Geometry check sheet. Reference: the model listing, model coordinates, mm. Face numbers are marked on the shaded views. A direction names the side the tool comes from. Round coordinates to 2 decimals unless told otherwise and drop trailing zeros. Order: outer loops, then holes, each group sorted by start corner. A loop starts at its lowest first (then second) coordinate and runs counter-clockwise, first axis right, second up. Notation, with made-up numbers: M 62.5,33.25 L 67.5,33.25 A18 ccw 67.5,64.25 Z; hole C -8,-18 d10. An arc over 180 degrees is marked long. Answer as a JSON object with one key per item and string values. Group by question number.
```python
from build123d import *
from build123d import SkipClean  # not in build123d's __all__

# Parameters (mm, degrees)
F0_W          = 151.5855640173
F0_H          = 149.6286615729
F1_DEPTH      = 11.684
F2_DEPTH      = 25.4
F3_W          = 4.1966233402
F3_H          = 25.7666455582
F3_W_2        = 24.8086545616
F3_H_2        = 24.7343285009
F3_W_3        = 8.3932466805
F3_H_3        = 20.2822238207
F3_W_4        = 29.5776501298
F3_H_4        = 8.4610134363
F5_DEPTH      = 25.4
F6_DEPTH      = 25.4
F8_W          = 13.618723955
F8_H          = 11.8162455037
F9_DEPTH      = 88.646
F10_W         = 90.7247327268
F10_H         = 75.9043544531
F11_DEPTH     = 13.97
F13_DEPTH     = 25.4
F14_DEPTH     = 125.476
F16_DEPTH     = 25.4
F17_R         = 4.969033059
F18_DEPTH     = 117.348
F20_DEPTH     = 87.376
F21_R         = 6.1087740457
F22_DEPTH     = 25.4
F23_DEPTH     = 25.4
F24_DEPTH     = 25.4
F25_R         = 5.08
F26_T1_DEPTH  = 44.704
F26_S5_W      = 5.08
F26_S5_H      = 5.08
F26_T6_DEPTH  = 5.08
F26_S11_W     = 5.08
F26_S11_H     = 5.08
F26_T12_DEPTH = 5.08
F27_W         = 27.1943286061
F27_H         = 16.5108405054
F28_DEPTH     = 61.722
F29_DEPTH     = 25.4
F30_DEPTH     = 160.02
F31_DEPTH     = 46.482


# Not quite as in the source:
# - a fillet or chamfer that OpenCascade refuses, or shapes differently, is made with other operations: its cross-section is extruded or revolved along the edge and cut away or added
# - after a boolean that leaves OpenCascade's solid faulty, fix() repairs it
# - a feature names something its author has since deleted; it is built from what else it names


with BuildPart() as f1:
    # F0 (on Top) → F1 (new body)
    with BuildSketch(Plane.XY):
        with Locations((1.5608146787, -0.5317740142)):
            Rectangle(F0_W, F0_H)
    extrude(amount=F1_DEPTH)

    # F2 (add): a face of the model
    f2_faces = [f1.faces().sort_by_distance(p)[0] for p in [
        (1.5608146787, -0.5317740142, 0),
    ]]
    extrude(f2_faces, amount=F2_DEPTH)

    # F3 (on face) → F5 (join)
    with BuildSketch(Plane(origin=(0, 0, -25.4), x_dir=(1, 0, 0), z_dir=(0, 0, -1))):
        with Locations((45.1576719061, 3.9362064563)):
            Rectangle(F3_W, F3_H)
        with Locations((-27.7178613469, -21.3142805733)):
            Rectangle(F3_W_2, F3_H_2)
        with Locations((47.2559835762, -43.8225567341)):
            Rectangle(F3_W_3, F3_H_3)
        with Locations((-54.0488772094, 67.9751783609)):
            Rectangle(F3_W_4, F3_H_4)
    extrude(amount=F5_DEPTH)

    # F6 (add): faces of the model
    f6_faces = [f1.faces().sort_by_distance(p)[0] for p in [
        (-54.0488772094, -67.9751783609, -50.8),
        (-27.7178613469, 21.3142805733, -50.8),
        (45.1576719061, -3.9362064563, -50.8),
        (47.2559835762, 43.8225567341, -50.8),
    ]]
    extrude(f6_faces, amount=F6_DEPTH)

    # F8 (on face) → F9 (join)
    with BuildSketch(Plane.XY.offset(11.684)):
        with Locations((-1.9266440067, -0.4005506635)):
            Rectangle(F8_W, F8_H)
    extrude(amount=F9_DEPTH)

    # F10 (on face) → F11 (join)
    with BuildSketch(Plane.XY.offset(100.33)):
        with Locations((-2.2270549089, -2.4033039808)):
            Rectangle(F10_W, F10_H)
    extrude(amount=F11_DEPTH)

    # F12 (on face) → F13 (join)
    with BuildSketch(Plane.XZ.offset(40.3554812074)):
        with BuildLine():
            ThreePointArc((-2.2270549227, 100.33), (2.7120859528, 102.3758591285), (4.7579450911, 107.315))
            ThreePointArc((4.7579450911, 107.315), (2.712085945, 112.2541408793), (-2.227054945, 114.3))
            ThreePointArc((-2.227054945, 114.3), (-9.2120549089, 107.3149999888), (-2.2270549227, 100.33))
        make_face()
    extrude(amount=F13_DEPTH)

    # F14 (add): a face of the model
    f14_faces = [f1.faces().sort_by_distance(p)[0] for p in [
        (-2.2270549089, -65.7554812074, 107.315),
    ]]
    with SkipClean():  # cleaning this boolean's faces spoils the solid; the shape is the same uncleaned
        extrude(f14_faces, amount=F14_DEPTH)

    # F15 (on face) → F16 (join)
    with BuildSketch(Plane.YZ.offset(43.1353114545)):
        with BuildLine():
            Line((-1.1355586467, 114.3), (1.1355586467, 114.3))
            ThreePointArc((1.1355586467, 114.3), (0, 114.4064722454), (-1.1355586467, 114.3))
        make_face()
        with BuildLine():
            ThreePointArc((-1.1355586467, 114.3), (-3.8974510358, 103.5937641266), (6.1087740457, 108.2976981997))
            ThreePointArc((6.1087740457, 108.2976981997), (4.7039340732, 112.1951492356), (1.1355586467, 114.3))
            Line((1.1355586467, 114.3), (-1.1355586467, 114.3))
        make_face()
    extrude(amount=F16_DEPTH)

    add(f1.part.fix(), mode=Mode.REPLACE)

    # F17 (on face) → F18 (join)
    with BuildSketch(Plane(origin=(0, 35.5488732457, 0), x_dir=(-1, 0, 0), z_dir=(0, 1, 0))):
        with Locations((0, 105.8959811926)):
            Circle(F17_R)
    extrude(amount=F18_DEPTH)

    # F19 (on face) → F20 (join)
    with BuildSketch(Plane(origin=(-47.5894212723, 0, 0), x_dir=(0, -1, 0), z_dir=(-1, 0, 0))):
        with BuildLine():
            Line((-3.5482673546, 114.3), (3.5482673546, 114.3))
            ThreePointArc((3.5482673546, 114.3), (0, 115.3617326707), (-3.5482673546, 114.3))
        make_face()
        with BuildLine():
            ThreePointArc((-3.5482673546, 114.3), (-3.0667012813, 103.2161631583), (6.4599488467, 108.901783824))
            ThreePointArc((6.4599488467, 108.901783824), (5.6856206657, 111.9684851053), (3.5482673546, 114.3))
            Line((3.5482673546, 114.3), (-3.5482673546, 114.3))
        make_face()
    extrude(amount=F20_DEPTH)

    # F21 (on face) → F22 (join)
    with BuildSketch(Plane.YZ.offset(68.5353114545)):
        with Locations((0, 108.2976981997)):
            Circle(F21_R)
    extrude(amount=F22_DEPTH)

    # F23 (add): faces of the model
    f23_faces = [f1.faces().sort_by_distance(p)[0] for p in [
        (0, 152.8968732457, 105.8959811926),
        (-2.2270549089, -191.2314812074, 107.315),
    ]]
    extrude(f23_faces, amount=F23_DEPTH, dir=(0, 1, 0))

    # F24 (add): a face of the model
    f24_faces = [f1.faces().sort_by_distance(p)[0] for p in [
        (93.9353114545, 0, 108.2976981997),
    ]]
    extrude(f24_faces, amount=F24_DEPTH)

    # F25
    f25_edges = [f1.edges().sort_by_distance(p)[0] for p in [
        (77.353597, -0.531774, 11.684),
        (1.560815, -75.346105, 11.684),
        (-74.231967, -0.531774, 11.684),
        (1.560815, 74.282557, 11.684),
        (77.353597, -75.346105, -6.858),
        (77.353597, 74.282557, -6.858),
        (77.353597, -0.531774, -25.4),
    ]]
    fillet(f25_edges, radius=F25_R)

    # F26: fillet of radius 5.08 on 2 edges, made by hand

    # F26_s2 → F26_t1 (cut)
    with BuildSketch(Plane.XY.offset(-38.1)):
        with BuildLine():
            ThreePointArc((-69.15196733, -75.3461048007), (-72.7440697784, -73.8582072491), (-74.23196733, -70.2661048007))
            Line((-74.23196733, -70.2661048007), (-74.23196733, -75.3461048007))
            Line((-74.23196733, -75.3461048007), (-69.15196733, -75.3461048007))
        make_face()
        with BuildLine():
            ThreePointArc((-69.15196733, 74.2825567722), (-72.7440697784, 72.7946592207), (-74.23196733, 69.2025567722))
            Line((-74.23196733, 69.2025567722), (-74.23196733, 74.2825567722))
            Line((-74.23196733, 74.2825567722), (-69.15196733, 74.2825567722))
        make_face()
    extrude(amount=F26_T1_DEPTH, mode=Mode.SUBTRACT)


with BuildPart() as f26_tool4:
    # F26_s5 → F26_t6 (new body)
    with BuildSketch(Plane.XZ.offset(-69.2025567722)):
        with Locations((-71.69196733, 9.144)):
            Rectangle(F26_S5_W, F26_S5_H)
    extrude(amount=-F26_T6_DEPTH)

    # F26_s7 → F26_t8 (revolve, cut)
    with BuildSketch(Plane(origin=(-69.15196733, 69.2025567722, 6.604), x_dir=(0.7071067812, 0, -0.7071067812), z_dir=(0.7071067812, 0, 0.7071067812))):
        with BuildLine():
            ThreePointArc((0, -5.08), (5.08, 0), (0, 5.08))
            Line((0, 5.08), (0, -5.08))
        make_face()
    revolve(axis=Axis((-69.15196733, 69.2025567722, 6.604), (0, 1, 0)), mode=Mode.SUBTRACT)


with BuildPart() as f1_1:
    add(f1.part, clean=False)

    # F26_t3: cut F26_tool4
    add(f26_tool4.part, mode=Mode.SUBTRACT)


with BuildPart() as f26_tool10:
    # F26_s11 → F26_t12 (new body)
    with BuildSketch(Plane.XZ.offset(70.2661048007)):
        with Locations((-71.69196733, 9.144)):
            Rectangle(F26_S11_W, F26_S11_H)
    extrude(amount=F26_T12_DEPTH)

    # F26_s13 → F26_t14 (revolve, cut)
    with BuildSketch(Plane(origin=(-69.15196733, -70.2661048007, 6.604), x_dir=(0.7071067812, 0, -0.7071067812), z_dir=(-0.7071067812, 0, -0.7071067812))):
        with BuildLine():
            ThreePointArc((0, -5.08), (5.08, 0), (0, 5.08))
            Line((0, 5.08), (0, -5.08))
        make_face()
    revolve(axis=Axis((-69.15196733, -70.2661048007, 6.604), (0, -1, 0)), mode=Mode.SUBTRACT)


with BuildPart() as f1_2:
    add(f1_1.part, clean=False)

    # F26_t9: cut F26_tool10
    add(f26_tool10.part, mode=Mode.SUBTRACT)

    # F27 (on face) → F28 (join)
    with BuildSketch(Plane(origin=(0, 0, -25.4), x_dir=(1, 0, 0), z_dir=(0, 0, -1))):
        with Locations((50.2156950533, 54.3001759797)):
            Rectangle(F27_W, F27_H)
    extrude(amount=F28_DEPTH)

    # F29 (add): a face of the model
    f29_faces = [f1_2.faces().sort_by_distance(p)[0] for p in [
        (119.3353114545, 0, 108.2976981997),
    ]]
    extrude(f29_faces, amount=F29_DEPTH)

    # F30 (add): a face of the model
    f30_faces = [f1_2.faces().sort_by_distance(p)[0] for p in [
        (144.7353114545, 0, 108.2976981997),
    ]]
    extrude(f30_faces, amount=F30_DEPTH)

    # F31 (add): a face of the model
    f31_faces = [f1_2.faces().sort_by_distance(p)[0] for p in [
        (-134.9654212723, 0, 108.901783824),
    ]]
    extrude(f31_faces, amount=F31_DEPTH)


solid = f1_2.part
```
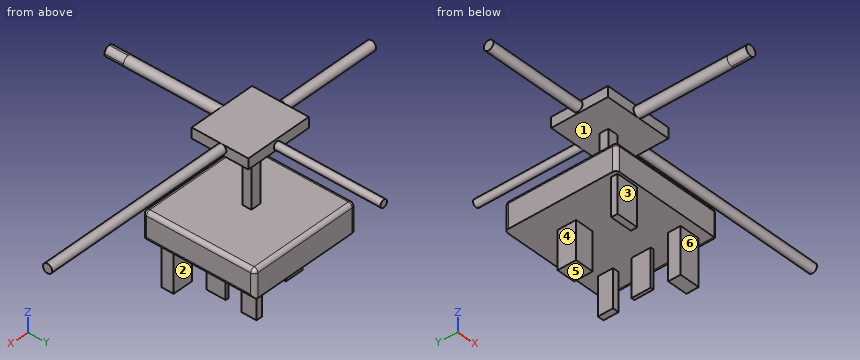
1) Release check for a two-part mould opening along Y. For the marked faces 1, 2 and 3 record: +Y half, -Y half, draft (parallel to the pull), parting line (faces both ways), or undercut.
2) Sectioned sample at B-B (y = -116.5). Record the boundary of the cut face in (x, z) (3 decimals), then the cut area to 3 significant figures.
3) Sectioned sample at C-C (z = 79). Record the boundary of the cut face in (x, y).
4) Go/stop test with flat-tipped pins: P1, Ø5, axis at y = -50.5, z = -71, coming from the -X side; P2, Ø8, axis at x = 32, z = 7, coming from the +Y side; P3, Ø22, axis at x = 51.5, z = -56.5, coming from the -Y side. Record where each tip stops, or that it passes through.
5) Thickness scan on line 1 along Z through (x, y) = (-2, -69.5); line 2 along Y through (x, z) = (-52.5, -48.5); line 3 along Z through (x, y) = (-146.5, -1). Record the ranges inside material, lowest first. Write a range as [from, to].
6) Sectioned sample at D-D (x = 198). Record the boundary of the cut face in (y, z), then the cut area to 3 significant figures.
7) Sectioned sample at A-A (z = -67.5). Record the boundary of the cut face in (x, y).
8) Set-up check for the marked faces 4, 5 and 6: record each of +Z, -Z, +X, -X, +Y, -Y from which the full face is reachable in a straight line by a thin tool's end or side.
Final values:
{
 "1": {"face 1": "draft", "face 2": "undercut", "face 3": "-Y half"},
 "2": {"outline": "C -2.227,107.315 d13.97", "area": "153 mm^2"},
 "3": {"outline": "M -8.74,-6.31 L 4.88,-6.31 L 4.88,5.51 L -8.74,5.51 Z"},
 "4": {"P1": "stops at x = 36.62", "P2": "stops at y = 74.28", "P3": "stops at y = -62.56"},
 "5": {"line 1": "z = [-25.4, 11.68], [100.33, 114.3]", "line 2": "y = [-72.21, -63.74]", "line 3": "z = [102.52, 115.28]"},
 "6": {"outline": "C 0,108.3 d12.22", "area": "117 mm^2"},
 "7": {"outline": "M -68.84,-72.21 L -39.26,-72.21 L -39.26,-63.74 L -68.84,-63.74 Z; M -40.12,8.95 L -15.31,8.95 L -15.31,33.68 L -40.12,33.68 Z; M 36.62,-62.56 L 63.81,-62.56 L 63.81,-46.04 L 36.62,-46.04 Z; M 43.06,-16.82 L 47.26,-16.82 L 47.26,8.95 L 43.06,8.95 Z; M 43.06,33.68 L 51.45,33.68 L 51.45,53.96 L 43.06,53.96 Z"},
 "8": {"face 4": "-Z, -X, +Y", "face 5": "-Z, +X, -X, +Y, -Y", "face 6": "-Z, +X, -X, -Y"}
}
